```python
from build123d import *

# Parameters (mm, degrees)
F0_R     = 9.525
F1_DEPTH = 15.875
F2_R     = 1.27


with BuildPart() as f1:
    # F0 (on Top) → F1 (new body)
    with BuildSketch(Plane.XY):
        with BuildLine():
            ThreePointArc((4.602905, 18.485556), (0, 16.51), (-4.602905, 18.485556))
            ThreePointArc((-4.602905, 18.485556), (-9.525, 16.497784), (-13.707508, 13.229011))
            ThreePointArc((-13.707508, 13.229011), (-14.298079, 8.255), (-18.310413, 5.256545))
            ThreePointArc((-18.310413, 5.256545), (-19.05, 0), (-18.310413, -5.256545))
            ThreePointArc((-18.310413, -5.256545), (-14.298079, -8.255), (-13.707508, -13.229011))
            ThreePointArc((-13.707508, -13.229011), (-9.525, -16.497784), (-4.602905, -18.485556))
            ThreePointArc((-4.602905, -18.485556), (0, -16.51), (4.602905, -18.485556))
            ThreePointArc((4.602905, -18.485556), (9.525, -16.497784), (13.707508, -13.229011))
            ThreePointArc((13.707508, -13.229011), (14.298079, -8.255), (18.310413, -5.256545))
            ThreePointArc((18.310413, -5.256545), (19.05, 0), (18.310413, 5.256545))
            ThreePointArc((18.310413, 5.256545), (14.298079, 8.255), (13.707508, 13.229011))
            ThreePointArc((13.707508, 13.229011), (9.525, 16.497784), (4.602905, 18.485556))
        make_face()
        Circle(F0_R, mode=Mode.SUBTRACT)
    extrude(amount=F1_DEPTH)

    # F2
    f2_edges = [f1.edges().sort_by_distance(p)[0] for p in [
        (13.707508, -13.229011, 7.9375),
        (4.602905, -18.485556, 7.9375),
        (18.310413, -5.256545, 7.9375),
        (18.310413, 5.256545, 7.9375),
        (13.707508, 13.229011, 7.9375),
        (4.602905, 18.485556, 7.9375),
        (-4.602905, 18.485556, 7.9375),
        (-13.707508, 13.229011, 7.9375),
        (-18.310413, 5.256545, 7.9375),
        (-18.310413, -5.256545, 7.9375),
        (-13.707508, -13.229011, 7.9375),
        (-4.602905, -18.485556, 7.9375),
    ]]
    fillet(f2_edges, radius=F2_R)


solid = f1.part
```
Read the model definition and answer for the solid it produces. Units are mm, in the model's axes. Give positions to 0.01 mm unless a question says otherwise; leave off trailing zeros. Order: outer loops, then holes, each group sorted by start corner. A loop starts at its lowest first (then second) coordinate and runs counter-clockwise, first axis right, second up. Notation, with made-up numbers: (39, -36.5) -> (95, -36.5) arc R21 ccw to (95, 1.5) -> close; hole circle Ø9 at (31.5, 20.5). An arc over 180 degrees is marked (long way). Write item = value, one per line.
1. A cutting plane is placed at A-A, the plane x = 0. Write down the section's boundary in (y, z) (3 decimals).
Numbers:
outline = (-16.51, 0) -> (-9.525, 0) -> (-9.525, 15.875) -> (-16.51, 15.875) -> close; (9.525, 0) -> (16.51, 0) -> (16.51, 15.875) -> (9.525, 15.875) -> close
2. A cutting plane is placed at B-B, the plane y = 0. Write down the section's boundary in (x, z) (3 decimals), and give its area (3 significant figures).
Numbers:
outline = (-19.05, 0) -> (-9.525, 0) -> (-9.525, 15.875) -> (-19.05, 15.875) -> close; (9.525, 0) -> (19.05, 0) -> (19.05, 15.875) -> (9.525, 15.875) -> close
area = 302 mm²
3. A cutting plane is placed at C-C, the plane x = -12.5. Write down the section's boundary in (y, z) (3 decimals).
Numbers:
outline = (-14.375, 0) -> (14.375, 0) -> (14.375, 15.875) -> (-14.375, 15.875) -> close
4. A cutting plane is placed at D-D, the plane y = 15. Write down the section's boundary in (x, z) (3 decimals).
Numbers:
outline = (-11.743, 0) -> (11.743, 0) -> (11.743, 15.875) -> (-11.743, 15.875) -> close
5. Given pin 1 (8 mm diameter, centred on y = -8.5, z = 2.5, fed in from +X); pin 2 (6 mm diameter, centred on y = -4, z = 10.5, fed in from +X); pin 3 (8 mm diameter, centred on x = -12.5, z = 9, fed in from -Y), each flat-ended and moving along its own axis, determine where each tip first touches the part or whether it passes through.
Numbers:
pin_1 = 18.51
pin_2 = 19.02
pin_3 = -17.05
6. Straight lines are drawn through the part: line 1 along X through (y, z) = (-2.5, 13); line 2 along Y through (x, z) = (-1, 2); line 3 along X through (y, z) = (5, 8.5). For each, find the intervals that lie inside material, in ascending order.
Numbers:
line_1 = -18.89 to -9.19, 9.19 to 18.89
line_2 = -16.59 to -9.47, 9.47 to 16.59
line_3 = -18.29 to -8.11, 8.11 to 18.29
7. The mould has two halves that part along Y. Classify faces 1 (the face through (14.267, -8.31, 7.826)), 2 (the face through (-9, -4, 0)), 3 (the face through (9.581, 16.466, 7.826)): +Y half, -Y half, draft (parallel to the pull), parting line (faces both ways), or undercut.
Numbers:
face_1 = undercut
face_2 = draft
face_3 = +Y half
